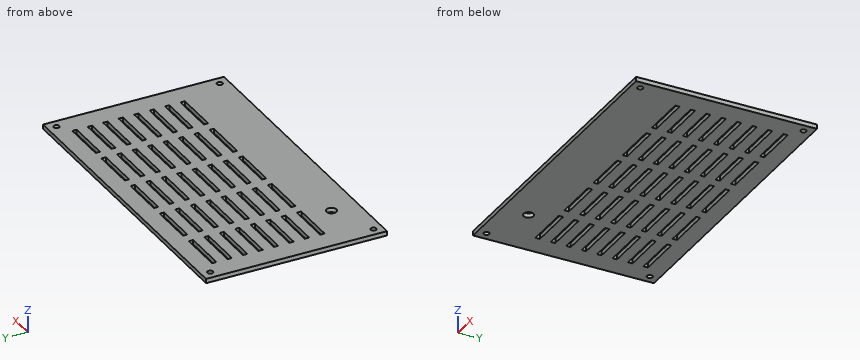
from build123d import *

# Parameters (mm, degrees)
SKETCH_W      = 140
SKETCH_H      = 82
PAD_DEPTH     = 2
SKETCH001_R   = 1.25
SKETCH001_R_2 = 2.25
SKETCH001_W   = 20
SKETCH001_H   = 2
POCKET_DEPTH  = 2


with BuildPart() as part:
    # Sketch → Pad (new body)
    with BuildSketch(Plane.XY):
        with Locations((70, 41)):
            Rectangle(SKETCH_W, SKETCH_H)
    extrude(amount=PAD_DEPTH)

    # Sketch001 (on Face6 of Pad) → Pocket (cut)
    with BuildSketch(Plane.XY.offset(2)):
        with Locations((4, 78)):
            Circle(SKETCH001_R)
        with Locations((136, 78)):
            Circle(SKETCH001_R)
        with Locations((136, 4)):
            Circle(SKETCH001_R)
        with Locations((4, 4)):
            Circle(SKETCH001_R)
        with Locations((25, 12)):
            Circle(SKETCH001_R_2)
        with Locations((20, 73)):
            Rectangle(SKETCH001_W, SKETCH001_H)
        with Locations((45, 73)):
            Rectangle(SKETCH001_W, SKETCH001_H)
        with Locations((70, 73)):
            Rectangle(SKETCH001_W, SKETCH001_H)
        with Locations((95, 73)):
            Rectangle(SKETCH001_W, SKETCH001_H)
        with Locations((120, 73)):
            Rectangle(SKETCH001_W, SKETCH001_H)
        with Locations((20, 66)):
            Rectangle(SKETCH001_W, SKETCH001_H)
        with Locations((45, 66)):
            Rectangle(SKETCH001_W, SKETCH001_H)
        with Locations((70, 66)):
            Rectangle(SKETCH001_W, SKETCH001_H)
        with Locations((95, 66)):
            Rectangle(SKETCH001_W, SKETCH001_H)
        with Locations((120, 66)):
            Rectangle(SKETCH001_W, SKETCH001_H)
        with Locations((20, 59)):
            Rectangle(SKETCH001_W, SKETCH001_H)
        with Locations((45, 59)):
            Rectangle(SKETCH001_W, SKETCH001_H)
        with Locations((70, 59)):
            Rectangle(SKETCH001_W, SKETCH001_H)
        with Locations((95, 59)):
            Rectangle(SKETCH001_W, SKETCH001_H)
        with Locations((120, 59)):
            Rectangle(SKETCH001_W, SKETCH001_H)
        with Locations((20, 52)):
            Rectangle(SKETCH001_W, SKETCH001_H)
        with Locations((45, 52)):
            Rectangle(SKETCH001_W, SKETCH001_H)
        with Locations((70, 52)):
            Rectangle(SKETCH001_W, SKETCH001_H)
        with Locations((95, 52)):
            Rectangle(SKETCH001_W, SKETCH001_H)
        with Locations((120, 52)):
            Rectangle(SKETCH001_W, SKETCH001_H)
        with Locations((20, 45)):
            Rectangle(SKETCH001_W, SKETCH001_H)
        with Locations((45, 45)):
            Rectangle(SKETCH001_W, SKETCH001_H)
        with Locations((70, 45)):
            Rectangle(SKETCH001_W, SKETCH001_H)
        with Locations((95, 45)):
            Rectangle(SKETCH001_W, SKETCH001_H)
        with Locations((120, 45)):
            Rectangle(SKETCH001_W, SKETCH001_H)
        with Locations((20, 38)):
            Rectangle(SKETCH001_W, SKETCH001_H)
        with Locations((45, 38)):
            Rectangle(SKETCH001_W, SKETCH001_H)
        with Locations((70, 38)):
            Rectangle(SKETCH001_W, SKETCH001_H)
        with Locations((95, 38)):
            Rectangle(SKETCH001_W, SKETCH001_H)
        with Locations((120, 38)):
            Rectangle(SKETCH001_W, SKETCH001_H)
        with Locations((20, 31)):
            Rectangle(SKETCH001_W, SKETCH001_H)
        with Locations((45, 31)):
            Rectangle(SKETCH001_W, SKETCH001_H)
        with Locations((70, 31)):
            Rectangle(SKETCH001_W, SKETCH001_H)
        with Locations((95, 31)):
            Rectangle(SKETCH001_W, SKETCH001_H)
        with Locations((120, 31)):
            Rectangle(SKETCH001_W, SKETCH001_H)
        with Locations((20, 24)):
            Rectangle(SKETCH001_W, SKETCH001_H)
        with Locations((45, 24)):
            Rectangle(SKETCH001_W, SKETCH001_H)
        with Locations((70, 24)):
            Rectangle(SKETCH001_W, SKETCH001_H)
        with Locations((95, 24)):
            Rectangle(SKETCH001_W, SKETCH001_H)
        with Locations((120, 24)):
            Rectangle(SKETCH001_W, SKETCH001_H)
    extrude(amount=-POCKET_DEPTH, mode=Mode.SUBTRACT)


solid = part.part
Verification items for the finished model (mm, model axes). Round coordinates to 2 decimals unless told otherwise and drop trailing zeros. Write each loop counter-clockwise with the first axis right and the second up, starting at its lowest first coordinate (ties: lowest second). Pieces come first, ordered by that corner, then holes.
(1) Depth check by flat-ended pin: pin 1 Ø3 at (x, y) = (69.5, 12) entering from -Z. Enter the tip coordinate at first touch or a pass-through.
Returned:
pin 1: stops at z = 0
(2) Material ranges on line 1 (Y direction, x = 4, z = 0.85); line 2 (X direction, y = 45.5, z = 1.35); line 3 (X direction, y = 78, z = 1.4), recorded low to high.
Returned:
line 1: y = 0 to 2.75, 5.25 to 76.75, 79.25 to 82
line 2: x = 0 to 10, 30 to 35, 55 to 60, 80 to 85, 105 to 110, 130 to 140
line 3: x = 0 to 2.75, 5.25 to 134.75, 137.25 to 140
(3) Section check A-A (y = 12). Enter the section's corners in (x, z).
Returned:
outline: (0, 0) - (22.75, 0) - (22.75, 2) - (0, 2) - close; (27.25, 0) - (140, 0) - (140, 2) - (27.25, 2) - close
(4) Section check B-B (x = 25). Give the number of separate pieces and of enclosed holes in the cut face, plus the area to 3 significant figures.
Returned:
separate pieces: 10
enclosed holes: 0
area: 123 mm2
